Part print with two shaded views. Sizes in mm from the minimum x, y, z corner. Give positions to 0.01 mm unless a question says otherwise; leave off trailing zeros. Write each loop counter-clockwise with the first axis right and the second up, starting at its lowest first coordinate (ties: lowest second). Pieces come first, ordered by that corner, then holes.
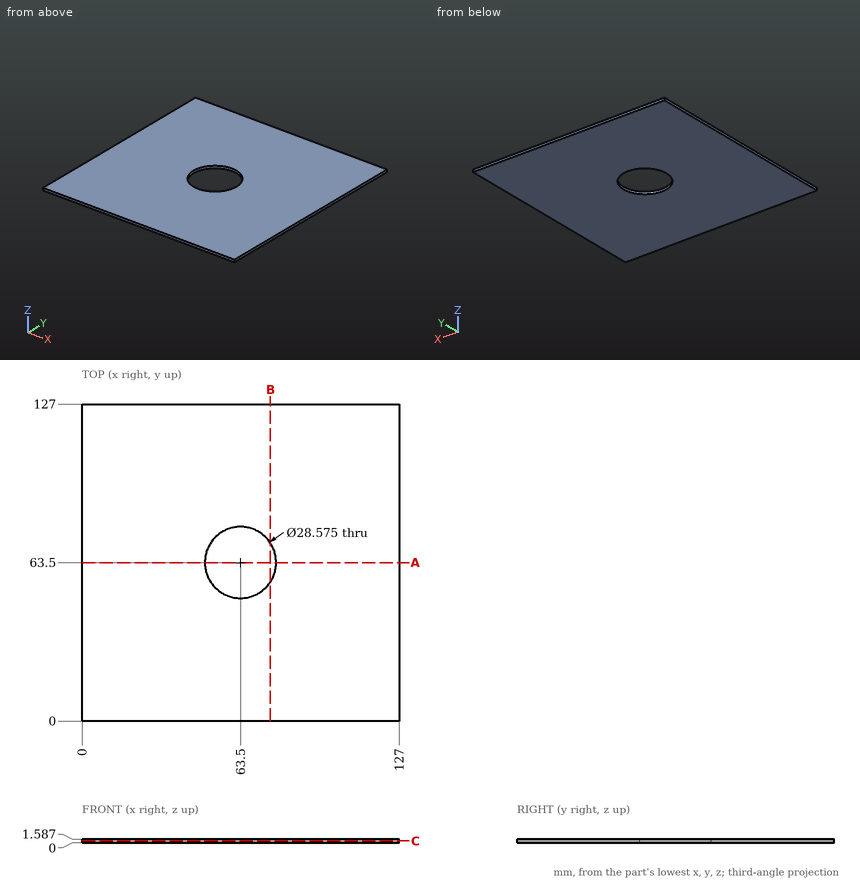
1) Flat gauge pin, fed straight in: P1, Ø17, axis at x = 63.5, y = 63.5, coming from the -Z side. Where does the tip first touch, or does it go through?
Check result:
P1: passes through
2) Saw through at C-C (z = 0.85). Write the cut outline in (x, y) (1 decimal), and give its area (3 significant figures).
Check result:
outline: (0, 0) - (127, 0) - (127, 127) - (0, 127) - close; hole circle Ø28.6 at (63.5, 63.5)
area: 15,500 mm2
3) Drill centre lines: L1, parallel to Y at x = 63.5, z = 0.95; L2, parallel to X at y = 53.5, z = 0.2 (1 decimal). Where is each one in solid material? Low to high.
Check result:
L1: y = 0 to 49.21, 77.79 to 127
L2: x = 0 to 53.3, 73.7 to 127
4) Saw through at B-B (x = 75.5). Write the cut outline in (y, z) (1 decimal), and give its area (3 significant figures).
Check result:
outline: (0, 0) - (55.7, 0) - (55.7, 1.6) - (0, 1.6) - close; (71.3, 0) - (127, 0) - (127, 1.6) - (71.3, 1.6) - close
area: 177 mm2
5) Saw through at A-A (y = 63.5). Write the cut outline in (x, z), and give its area (3 significant figures).
Check result:
outline: (0, 0) - (49.21, 0) - (49.21, 1.59) - (0, 1.59) - close; (77.79, 0) - (127, 0) - (127, 1.59) - (77.79, 1.59) - close
area: 156 mm2
